Study the drawing (mm; zero at the part's minimum x, y, z) and answer. A direction names the side the tool comes from. Give positions to 0.01 mm unless a question says otherwise; leave off trailing zeros. Order: outer loops, then holes, each group sorted by start corner. A loop starts at its lowest first (then second) coordinate and runs counter-clockwise, first axis right, second up.
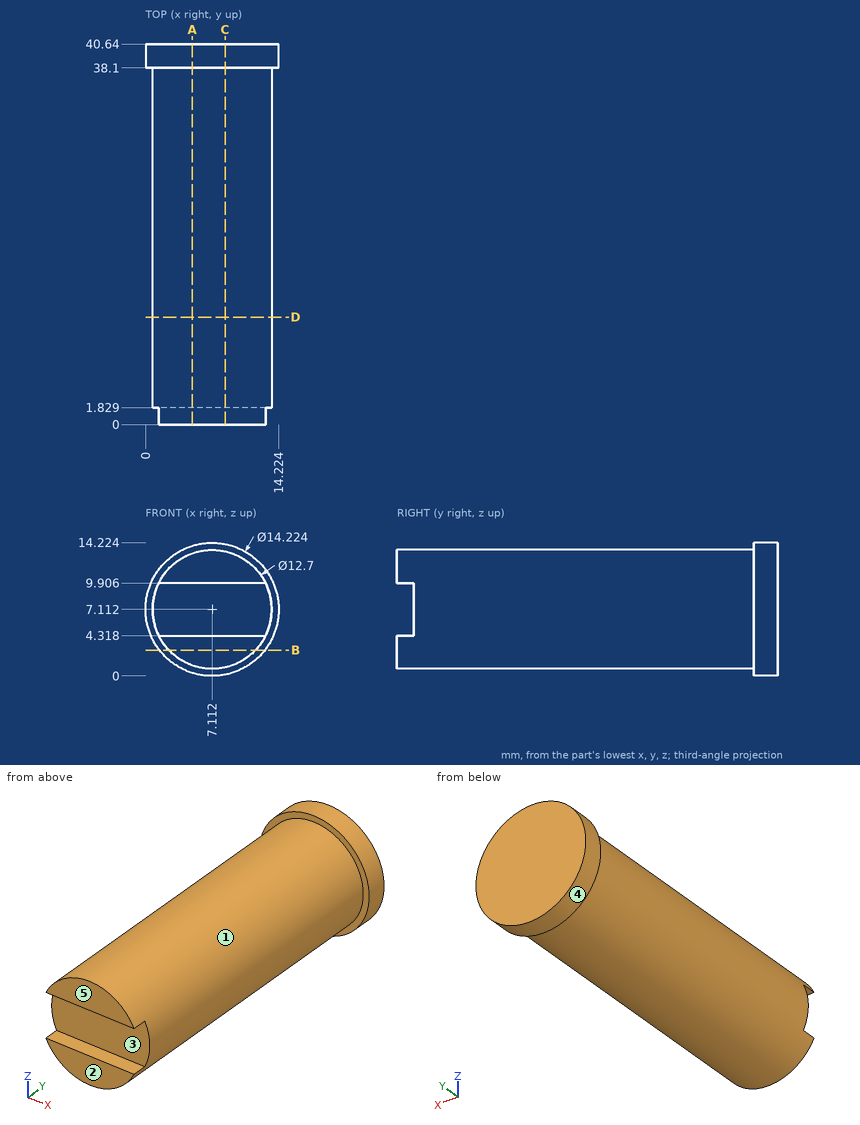
1) Find section B-B (z = 2.75). Write down the section's boundary in (x, y) (1 decimal), then the cut area to 3 significant figures.
Geometry says:
outline: (1.5, 38.1) - (2.5, 38.1) - (2.5, 0) - (11.7, 0) - (11.7, 38.1) - (12.7, 38.1) - (12.7, 40.6) - (1.5, 40.6) - close
area: 380 mm2
2) Find section A-A (x = 5). Write down the section's boundary in (y, z).
Geometry says:
outline: (0, 1.12) - (38.1, 1.12) - (38.1, 0.32) - (40.64, 0.32) - (40.64, 13.9) - (38.1, 13.9) - (38.1, 13.1) - (0, 13.1) - (0, 9.91) - (1.83, 9.91) - (1.83, 4.32) - (0, 4.32) - close
3) Given P1, Ø0.9, axis at x = 5.5, y = 1, coming from the -Z side; P2, Ø2, axis at x = 12, y = 15, coming from the -Z side; P3, Ø8, axis at y = 26.5, z = 4.5, coming from the -X side, each flat-ended and moving along its own axis, determine where each tip first touches the part or whether it passes through.
Geometry says:
P1: stops at z = 0.87
P2: stops at z = 2.09
P3: stops at x = 0.76
4) Find section C-C (x = 8.5). Write down the section's boundary in (y, z).
Geometry says:
outline: (0, 0.92) - (38.1, 0.92) - (38.1, 0.14) - (40.64, 0.14) - (40.64, 14.09) - (38.1, 14.09) - (38.1, 13.31) - (0, 13.31) - (0, 9.91) - (1.83, 9.91) - (1.83, 4.32) - (0, 4.32) - close
5) Straight lines are drawn through the part: probe 1 along Y at (x, z) = (6, 8.75); probe 2 along Y at (x, z) = (4.25, 13.25); probe 3 along Z at (x, y) = (7.25, 29.5). For each, find the intervals that lie inside material, in ascending order.
Geometry says:
probe 1: y = 1.83 to 40.64
probe 2: y = 38.1 to 40.64
probe 3: z = 0.76 to 13.46
6) For a pull along Z with two mould halves and no side action, classify the marked faces 3, 4 and 5 as +Z half, -Z half, draft (parallel to the pull), parting line (faces both ways), or undercut.
Geometry says:
face 3: undercut
face 4: parting line
face 5: draft
7) A tool of negligible diameter and unlimited length cuts with its end or side. For the marked faces 1 and 2, from which of +Z, -Z, +X, -X, +Y, -Y can it reach the whole face along a straight path? Write none if from no direction.
Geometry says:
face 1: -Y
face 2: +Z, -Z, +X, -X, -Y
8) Find section D-D (y = 11.5). Write down the section's boundary in (x, z), then the cut area to 3 significant figures.
Geometry says:
outline: circle Ø12.7 at (7.11, 7.11)
area: 127 mm2
